Verification items for the finished model (mm, model axes). A direction names the side the tool comes from. Give positions to 0.01 mm unless a question says otherwise; leave off trailing zeros. Write each loop counter-clockwise with the first axis right and the second up, starting at its lowest first coordinate (ties: lowest second). Pieces come first, ordered by that corner, then holes.
from build123d import *

# Parameters (mm, degrees)
SKETCH2_R               = 18.5
BOSS_EXTRUDE1_DEPTH     = 26
SKETCH3_R               = 17.738120084
BOSS_EXTRUDE2_DEPTH     = 50
SKETCH4_R               = 1.585
BOSS_EXTRUDE3_DEPTH     = 19.5
SKETCH5_R               = 6
BOSS_EXTRUDE4_DEPTH     = 5.5
SKETCH6_R               = 3
BOSS_EXTRUDE5_DEPTH     = 16.5
CUT_EXTRUDE1_DEPTH      = 121.377531126
CUT_EXTRUDE1_DEPTH_BACK = 12


with BuildPart() as part:
    # Sketch2 → Boss-Extrude1 (new body)
    with BuildSketch(Plane.XY):
        with Locations(Location((0, 0, 0), (0, 0, 180))):
            Circle(SKETCH2_R)
    extrude(amount=BOSS_EXTRUDE1_DEPTH)

    # Sketch3 → Boss-Extrude2 (add)
    with BuildSketch(Plane.XY.offset(26)):
        Circle(SKETCH3_R)
    extrude(amount=BOSS_EXTRUDE2_DEPTH)

    # Sketch4 → Boss-Extrude3 (add)
    with BuildSketch(Plane.XY.offset(76)):
        Circle(SKETCH4_R)
    extrude(amount=BOSS_EXTRUDE3_DEPTH)

    # Sketch5 → Boss-Extrude4 (add)
    with BuildSketch(Plane(origin=(0, 0, 0), x_dir=(-1, 0, 0), z_dir=(0, 0, -1))):
        with Locations(Location((0, 7, 0), (0, 0, 180))):
            Circle(SKETCH5_R)
    extrude(amount=BOSS_EXTRUDE4_DEPTH)

    # Sketch6 → Boss-Extrude5 (add)
    with BuildSketch(Plane(origin=(0, 0, -5.5), x_dir=(-1, 0, 0), z_dir=(0, 0, -1))):
        with Locations((0, 7)):
            Circle(SKETCH6_R)
    extrude(amount=BOSS_EXTRUDE5_DEPTH)

    # Sketch7 → Cut-Extrude1 (cut, two sides: drawn at the far end of the back side and taken through both)
    with BuildSketch(Plane(origin=(0, 0, -22), x_dir=(-1, 0, 0), z_dir=(0, 0, -1)).offset(-CUT_EXTRUDE1_DEPTH_BACK)):
        with BuildLine():
            ThreePointArc((1.198957881, 9.75), (0, 10), (-1.198957881, 9.75))
            Line((-1.198957881, 9.75), (1.198957881, 9.75))
        make_face()
    extrude(amount=CUT_EXTRUDE1_DEPTH + CUT_EXTRUDE1_DEPTH_BACK, mode=Mode.SUBTRACT)


solid = part.part
Item 1: Depth check by flat-ended pin: pin 1 (2 mm diameter, centred on x = 3.5, y = 12.5, fed in from +Z); pin 2 (6 mm diameter, centred on y = -12.5, z = 71, fed in from -X); pin 3 (10 mm diameter, centred on x = -9.5, z = 60.5, fed in from -Y). Enter the tip coordinate at first touch or a pass-through.
Answer key:
pin 1: stops at z = 76
pin 2: stops at x = -14.98
pin 3: stops at y = -17.16
Item 2: Sectioned sample at B-B on y = 8.5. Record the cut outline in (x, z), then the cut area to 3 significant figures.
Answer key:
outline: (-16.43, 0) - (-5.81, 0) - (-5.81, -5.5) - (-2.6, -5.5) - (-2.6, -22) - (2.6, -22) - (2.6, -5.5) - (5.81, -5.5) - (5.81, 0) - (16.43, 0) - (16.43, 26) - (15.57, 26) - (15.57, 76) - (-15.57, 76) - (-15.57, 26) - (-16.43, 26) - close
area: 2,560 mm2
Item 3: Scan lines: line 1 along Z through (x, y) = (-7, 5); line 2 along Y through (x, z) = (-0.5, 45); line 3 along Z through (x, y) = (10.5, -14.5). Record each from-to range of solid material in increasing order.
Answer key:
line 1: z = 0 to 76
line 2: y = -17.73 to 17.73
line 3: z = 0 to 26
Item 4: Sectioned sample at D-D on x = -16. Record the cut outline in (y, z), then the cut area to 3 significant figures.
Answer key:
outline: (-9.29, 0) - (9.29, 0) - (9.29, 26) - (7.66, 26) - (7.66, 76) - (-7.66, 76) - (-7.66, 26) - (-9.29, 26) - close
area: 1,250 mm2
Item 5: Sectioned sample at A-A on x = 0. Record the cut outline in (y, z) (3 decimals).
Answer key:
outline: (-18.5, 0) - (1, 0) - (1, -5.5) - (4, -5.5) - (4, -22) - (9.75, -22) - (9.75, -10) - (10, -10) - (10, -5.5) - (13, -5.5) - (13, 0) - (18.5, 0) - (18.5, 26) - (17.738, 26) - (17.738, 76) - (1.585, 76) - (1.585, 95.5) - (-1.585, 95.5) - (-1.585, 76) - (-17.738, 76) - (-17.738, 26) - (-18.5, 26) - close
Item 6: Set-up check for faces 1 (the face through (-15, 10, 26)), 2 (the face through (-3, 8, -5.5)), 3 (the face through (0, 9.75, -16)), 4 (the face through (0, 0, 95.5)): record each of +Z, -Z, +X, -X, +Y, -Y from which the full face is reachable in a straight line by a thin tool's end or side.
Answer key:
face 1: +Z
face 2: -Z
face 3: -Z, +X, -X, +Y
face 4: +Z, +X, -X, +Y, -Y
Item 7: Sectioned sample at C-C on z = 3. Record the cut outline in (x, y), then the cut area to 3 significant figures.
Answer key:
outline: circle Ø37 at (0, 0)
area: 1,080 mm2
